Source: three-view drawing plus pictorial views. Frame: mm from the lowest corner of the part. A direction names the side the tool comes from. Round coordinates to 2 decimals unless told otherwise and drop trailing zeros. Loops run counter-clockwise (first coordinate to the right, second up) from the corner with the lowest first, then second, coordinate; pieces in that order, holes last. Notation, with made-up numbers: M 78,49.25 L 99,49.25 A22 cw 99,85.25 Z; hole C 81,-2 d6. An arc over 180 degrees is marked long. Return JSON: item names as keys, results as strings. Group by question number.
1) Section B-B (y = 12.5). Output: boundary loops of the cut face in (x, z).
2) Mould query, pull axis X, two halves, no side actions, for the marked faces 1, 2 and 3. Classes: +X half, -X half, draft (parallel to the pull), parting line (faces both ways), or undercut.
3) Access query for the marked faces 4, 5 and 6. Directions: +Z, -Z, +X, -X, +Y, -Y. A direction counts if a zero-diameter tool reaches every point of the face in a straight line with its end or side. Return the directions, or none.
4) Material intervals for line 1 (Y direction, x = 15.5, z = 20.5); line 2 (X direction, y = 13, z = 27); line 3 (X direction, y = 26.8, z = 22.5), sorted ascending. Write a range as from..to.
5) Section A-A (z = 45). Output: boundary loops of the cut face in (x, y).
6) Section D-D (z = 34). Output: boundary loops of the cut face in (x, y), plus the area to 3 significant figures.
7) Contact query for flat-ended pins moving along their axis: P1, Ø10.5, axis at x = 15, y = 13, coming from the -Z side; P2, Ø1.9, axis at x = 15, z = 22.5, coming from the +Y side; P3, Ø3.5, axis at x = 15, z = 7.5, coming from the +Y side; P4, Ø3, axis at x = 12, y = 37.5, coming from the -Z side. Output: stop coordinate, or through.
8) Section C-C (z = 15). Output: boundary loops of the cut face in (x, y), plus the area to 3 significant figures.
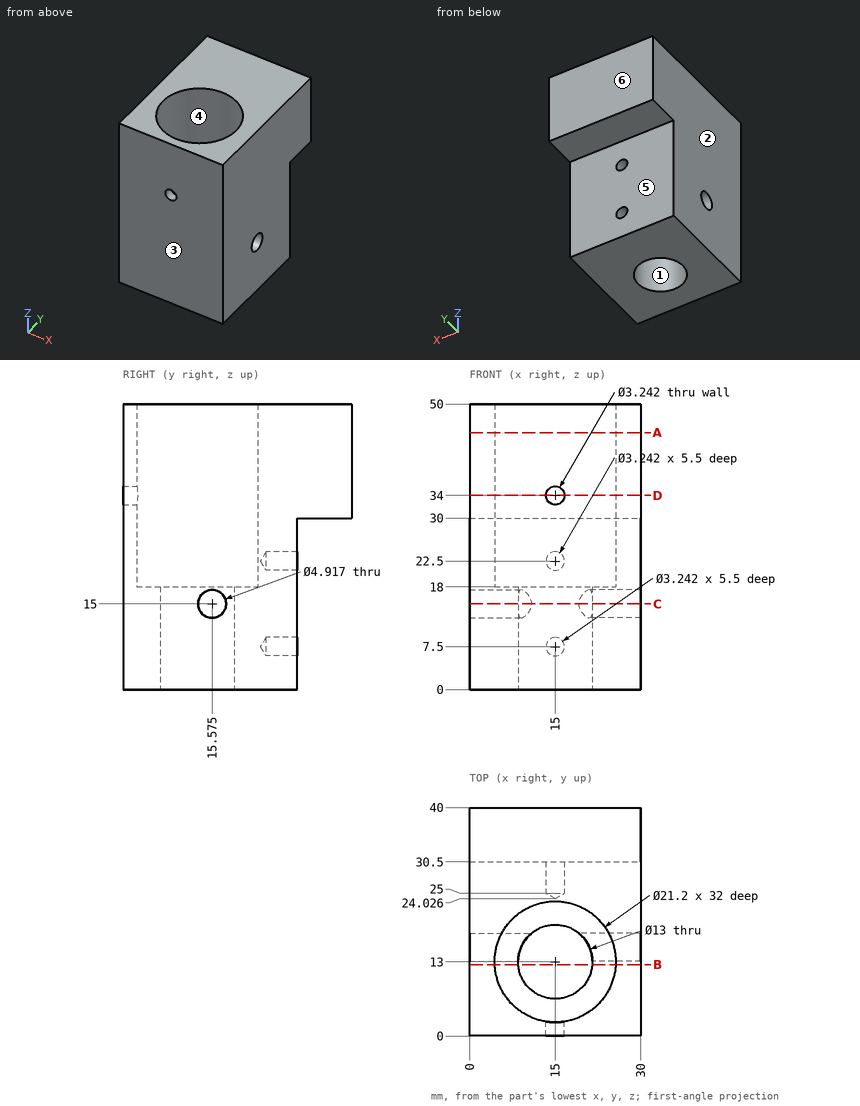
Returned:
{
 "1": {"outline": "M 0,0 L 8.52,0 L 8.52,18 L 4.41,18 L 4.41,50 L 0,50 Z; M 21.48,0 L 30,0 L 30,50 L 25.59,50 L 25.59,18 L 21.48,18 Z"},
 "2": {"face 1": "undercut", "face 2": "-X half", "face 3": "draft"},
 "3": {"face 4": "+Z", "face 5": "-Z, +X, -X, +Y", "face 6": "+Z, -Z, +X, -X, +Y"},
 "4": {"line 1": "y = 0..2.41, 23.59..30.5", "line 2": "x = 0..4.4, 25.6..30", "line 3": "x = 0..13.38, 16.62..30"},
 "5": {"outline": "M 0,0 L 30,0 L 30,40 L 0,40 Z; hole C 15,13 d21.2"},
 "6": {"outline": "M 0,0 L 13.38,0 L 13.38,2.52 A10.6 cw long 16.62,2.52 L 16.62,0 L 30,0 L 30,40 L 0,40 Z", "area": "839 mm^2"},
 "7": {"P1": "passes through", "P2": "stops at y = 24.6", "P3": "stops at y = 30.5", "P4": "stops at z = 30"},
 "8": {"outline": "M 0,0 L 30,0 L 30,13.12 L 21.5,13.12 A6.5 cw long 8.5,13.12 L 0,13.12 Z; M 0,18.03 L 10.89,18.03 A6.5 cw 19.11,18.03 L 30,18.03 L 30,30.5 L 0,30.5 Z", "area": "691 mm^2"}
}
